For this review, take the finished solid that the model builds, in its own axes (mm). A direction names the side the tool comes from. Coordinates: 2 decimals unless noted, no trailing zeros. Order: outer loops, then holes, each group sorted by start corner. A loop starts at its lowest first (then second) coordinate and runs counter-clockwise, first axis right, second up. Notation, with made-up numbers: (88.5, -5) -> (107.5, -5) arc R17 cw to (107.5, 2) -> close; hole circle Ø7 at (58, -24.5). An arc over 180 degrees is marked (long way). Write item = value, one per line. Start each with the question number.
1) Wall thickness on probe 1 along X at (y, z) = (-1.7, -1); probe 2 along Y at (x, z) = (0.1, -33): over which ranges is each line inside the solid? List them lowest first. Write a range as [from, to].
2) Insertion check: pin 1 Ø1.2 at (x, z) = (-1.5, -3.5) entering from -Y; pin 2 Ø1.2 at (x, z) = (-2, -17.5) entering from +Y; pin 3 Ø0.7 at (y, z) = (1.5, 2) entering from +X. Each pin has a flat end and moves straight along its axis. Give the tip position at first contact, or say it passes through.
3) Consider section A-A on z = 7. Give the boundary of the cut face in (x, y), and give its area (3 significant figures).
4) Machinability: for faces 1 (the face through (0.8, -2, -1)), 2 (the face through (-0.8, -2, -1)), 3 (the face through (-2, 0.8, -1)), 4 (the face through (0.8, 2, -1)), which of the approach directions +Z, -Z, +X, -X, +Y, -Y give a long, thin tool a straight path to every point of the face, cutting with its end or side? Answer none if there is none.
Autodesk Inventor part; units mm, degrees
ref_plane "YZ Plane" through (0, 0, 0) normal (1, 0, 0) x (0, 1, 0)
ref_plane "XZ Plane" through (0, 0, 0) normal (0, 1, 0) x (-1, 0, 0)
ref_plane "XY Plane" through (0, 0, 0) normal (0, 0, 1) x (1, 0, 0)
sketch "Sketch1" plane through (0, 0, 0) normal (0, 0, 1) x (1, 0, 0)
  circle A0 centre (0, 0) radius 2.4 construction
  line L0 (-0.8, 2.2627) -> (-0.8, 0.8)
  line L1 (-0.8, 0.8) -> (-2.2627, 0.8)
  line L2 (-2.2627, -0.8) -> (-0.8, -0.8)
  line L3 (-0.8, -0.8) -> (-0.8, -2.2627)
  line L4 (0.8, -2.2627) -> (0.8, -0.8)
  line L5 (0.8, -0.8) -> (2.2627, -0.8)
  line L6 (2.2627, 0.8) -> (0.8, 0.8)
  line L7 (0.8, 0.8) -> (0.8, 2.2627)
  arc A1 (0.8, 2.2627) -> (-0.8, 2.2627) centre (0, 0) ccw
  arc A2 (-2.2627, 0.8) -> (-2.2627, -0.8) centre (0, 0) ccw
  arc A3 (-0.8, -2.2627) -> (0.8, -2.2627) centre (0, 0) ccw
  arc A4 (2.2627, -0.8) -> (2.2627, 0.8) centre (0, 0) ccw
  dimension "d0" = 4.8
  dimension "d1" = 1.6
extrude "Extrusion1" add sketch "Sketch1" along normal mid plane 88
fillet "Fillet1" radius 0.4 8 edges at (0, 2.4, 44) (-2.4, 0, 44) (0, -2.4, 44) (2.4, 0, 44) (2.4, 0, -44) (0, 2.4, -44) (-2.4, 0, -44) (0, -2.4, -44)
equation "\"d0\" = kd"
equation "\"d1\" = axlet"
equation "\"d2\" = 11 * lu"
equation "\"d4\" = tf"
equation "\"unit\" = 8"
properties part number "23948-Yellow" material "ABS Plastic"
Answer sheet:
q1.probe_1 = [-0.8, 0.8]
q1.probe_2 = [-2.4, 2.4]
q2.pin_1 = -0.8
q2.pin_2 = 0.8
q2.pin_3 = 0.8
q3.outline = (-2.26, -0.8) -> (-0.8, -0.8) -> (-0.8, -2.26) arc R2.4 ccw to (0.8, -2.26) -> (0.8, -0.8) -> (2.26, -0.8) arc R2.4 ccw to (2.26, 0.8) -> (0.8, 0.8) -> (0.8, 2.26) arc R2.4 ccw to (-0.8, 2.26) -> (-0.8, 0.8) -> (-2.26, 0.8) arc R2.4 ccw to start
q3.area = 12.5 mm2
q4.face_1 = +Z, -Z, +X, -Y
q4.face_2 = +Z, -Z, -X, -Y
q4.face_3 = +Z, -Z, -X, +Y
q4.face_4 = +Z, -Z, +X, +Y
